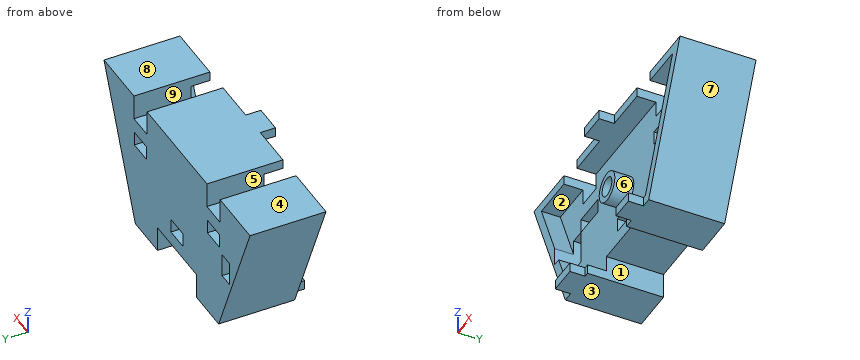
Autodesk Inventor part; units mm, degrees
ref_plane "YZ Plane" through (0, 0, 0) normal (1, 0, 0) x (0, 1, 0)
ref_plane "XZ Plane" through (0, 0, 0) normal (0, 1, 0) x (-1, 0, 0)
ref_plane "XY Plane" through (0, 0, 0) normal (0, 0, 1) x (1, 0, 0)
sketch "Sketch1" plane through (0, 0, 0) normal (0, 1, 0) x (-1, 0, 0)
  line L0 (-15, 7.5) -> (15, 7.5)
  line L1 (15, 7.5) -> (15, -7.5)
  line L2 (15, -7.5) -> (-15, -7.5)
  line L3 (-15, -7.5) -> (-15, 7.5)
  line L4 (-15, 7.5) -> (15, -7.5) construction
  line L5 (15, 7.5) -> (-15, -7.5) construction
  point P0 (0, 0)
  dimension "d0" = 30
  dimension "d1" = 15
extrude "Extrusion1" add sketch "Sketch1" along normal blind 8
sketch "Sketch3" plane through (0, 8, 0) normal (0, 1, 0) x (1, 0, 0)
  line L0 (-15, 7.5) -> (-15, -7.5)
  line L1 (-15, -7.5) -> (15, -7.5)
  line L2 (-15, -7.5) -> (15, -7.5)
  line L3 (15, -7.5) -> (8.5, 7.6369)
  line L4 (-15, -7.5) -> (-8.5, 7.6369)
  line L5 (-8.5, 7.6369) -> (8.5, 7.6369)
  line L6 (-10.75, -1.2417) -> (-9.25, -1.2417)
  line L7 (-9.25, -1.2417) -> (-9.25, 1.2583)
  line L8 (-9.25, 1.2583) -> (-10.75, 1.2583)
  line L9 (-10.75, 1.2583) -> (-10.75, -1.2417)
  line L10 (-10.75, -1.2417) -> (-9.25, 1.2583) construction
  line L11 (-9.25, -1.2417) -> (-10.75, 1.2583) construction
  line L12 (-6.25, -3.25) -> (-8.75, -3.25)
  line L13 (-8.75, -3.25) -> (-8.75, -1.75)
  line L14 (-8.75, -1.75) -> (-6.25, -1.75)
  line L15 (-6.25, -1.75) -> (-6.25, -3.25)
  line L16 (-6.25, -3.25) -> (-8.75, -1.75) construction
  line L17 (-8.75, -3.25) -> (-6.25, -1.75) construction
  line L18 (8.75, -1.75) -> (6.25, -1.75)
  line L19 (6.25, -1.75) -> (6.25, -3.25)
  line L20 (6.25, -3.25) -> (8.75, -3.25)
  line L21 (8.75, -3.25) -> (8.75, -1.75)
  line L22 (8.75, -1.75) -> (6.25, -3.25) construction
  line L23 (6.25, -1.75) -> (8.75, -3.25) construction
  line L24 (15, 7.5) -> (-15, 7.5)
  line L25 (-15, -7.5) -> (-15, 7.5)
  line L26 (-15, 7.5) -> (15, 7.5)
  line L27 (15, 7.5) -> (15, -7.5)
  line L28 (1.25, 1.8869) -> (-1.25, 1.8869)
  line L29 (-1.25, 1.8869) -> (-1.25, 3.3869)
  line L30 (-1.25, 3.3869) -> (1.25, 3.3869)
  line L31 (1.25, 3.3869) -> (1.25, 1.8869)
  line L32 (1.25, 1.8869) -> (-1.25, 3.3869) construction
  line L33 (-1.25, 1.8869) -> (1.25, 3.3869) construction
  point P0 (0, 0)
  point P1 (-10, 0.0083)
  point P2 (-7.5, -2.5)
  point P3 (7.5, -2.5)
  point P4 (0, -7.5)
  point P5 (0, -7.5)
  point P6 (0, 2.6369)
  point P7 (8.5588, 7.5)
  point P8 (-8.5588, 7.5)
  dimension "d19" = 17
  dimension "d20" = 1.5
  dimension "d21" = 2.5
  dimension "d22" = 5
  dimension "d24" = 7.5
  dimension "d25" = 7.5
  dimension "d26" = 5
  dimension "d27" = 5
  dimension "d28" = 5
  dimension "d29" = 0
extrude "Extrusion3" cut sketch "Sketch3" against normal blind 8 contours L24 L4 L0 | L3 L24 L27 | L9 L8 L7 L6 | L12 L13 L14 L15 | L21 L20 L19 L18 | L28 L29 L30 L31
sketch "Sketch4" plane through (0, 0, 0) normal (0, -1, 0) x (1, 0, 0)
  line L0 (-9.25, 1.7417) -> (-10.75, 1.7417)
  line L1 (-10.75, 1.7417) -> (-10.75, -1.7583)
  line L2 (-10.75, -1.7583) -> (-9.25, -1.7583)
  line L3 (-9.25, -1.7583) -> (-9.25, 1.7417)
  line L4 (-9.25, 1.7417) -> (-10.75, -1.7583) construction
  line L5 (-10.75, 1.7417) -> (-9.25, -1.7583) construction
  line L6 (-10.75, -1.2583) -> (-10.75, 1.2417)
  line L7 (-9.25, 1.2417) -> (-9.25, -1.2583)
  line L8 (-9.25, -1.2583) -> (-10.75, -1.2583)
  line L9 (-10.75, 1.2417) -> (-9.25, 1.2417)
  line L10 (-8.75, 3.25) -> (-6.25, 3.25) construction
  line L11 (-7.5, 3.25) -> (-7.5, 1.75) construction
  line L12 (-8.75, 1.75) -> (-6.25, 1.75) construction
  line L13 (-1.25, -1.8869) -> (1.25, -1.8869) construction
  line L14 (0, -1.8869) -> (0, -3.3869) construction
  line L15 (1.25, -3.3869) -> (-1.25, -3.3869) construction
  line L16 (6.25, 3.25) -> (8.75, 3.25) construction
  line L17 (7.5, 3.25) -> (7.5, 1.75) construction
  line L18 (8.75, 1.75) -> (6.25, 1.75) construction
  line L19 (9.25, 3.25) -> (5.75, 3.25)
  line L20 (5.75, 3.25) -> (5.75, 1.75)
  line L21 (5.75, 1.75) -> (9.25, 1.75)
  line L22 (9.25, 1.75) -> (9.25, 3.25)
  line L23 (9.25, 3.25) -> (5.75, 1.75) construction
  line L24 (5.75, 3.25) -> (9.25, 1.75) construction
  line L25 (1.75, -1.8869) -> (-1.75, -1.8869)
  line L26 (-1.75, -1.8869) -> (-1.75, -3.3869)
  line L27 (-1.75, -3.3869) -> (1.75, -3.3869)
  line L28 (1.75, -3.3869) -> (1.75, -1.8869)
  line L29 (1.75, -1.8869) -> (-1.75, -3.3869) construction
  line L30 (-1.75, -1.8869) -> (1.75, -3.3869) construction
  line L31 (-5.75, 3.25) -> (-9.25, 3.25)
  line L32 (-9.25, 3.25) -> (-9.25, 1.75)
  line L33 (-9.25, 1.75) -> (-5.75, 1.75)
  line L34 (-5.75, 1.75) -> (-5.75, 3.25)
  line L35 (-5.75, 3.25) -> (-9.25, 1.75) construction
  line L36 (-9.25, 3.25) -> (-5.75, 1.75) construction
  point P0 (0, 0)
  point P1 (-10, -0.0083)
  point P2 (7.5, 2.5)
  point P3 (0, -2.6369)
  point P4 (-7.5, 2.5)
  point P5 (-10.75, 1.2417)
  dimension "d32" = 0
  dimension "d33" = 0
  dimension "d34" = 0.5
  dimension "d35" = 0.5
  dimension "d36" = 3.5
  dimension "d37" = 3.5
  dimension "d38" = 3.5
extrude "Extrusion4" cut sketch "Sketch4" against normal blind 3.5
sketch "Sketch5" plane through (0, 0, 0) normal (0, -1, 0) x (1, 0, 0)
  line L0 (-9.25, -1.7583) -> (-10.75, -1.7583)
  line L1 (-15, 7.5) -> (-8.5588, -7.5)
  line L2 (8.5588, -7.5) -> (-8.5588, -7.5)
  line L3 (-7.8999, -6.5) -> (7.8999, -6.5)
  line L4 (7.8999, -6.5) -> (13.4823, 6.5)
  line L5 (8.5588, -7.5) -> (15, 7.5)
  line L6 (-15, 7.5) -> (15, 7.5)
  line L7 (13.4823, 6.5) -> (-14, 6.5)
  line L8 (-7.8999, -6.5) -> (-13.4823, 6.5)
  point P0 (0, 0)
  point P1 (-13.4823, 6.5)
  dimension "d41" = 1
  dimension "d42" = 1
  dimension "d43" = 1
  dimension "d44" = 1
  dimension "d45" = 1
  dimension "d46" = 1
sketch "Sketch2" plane through (0, 8, 0) normal (0, 1, 0) x (1, 0, 0)
  line L0 (4, 7.5) -> (-4, 7.5)
  line L1 (-4, 7.5) -> (-4, 4.8)
  line L2 (-4, 4.8) -> (4, 4.8)
  line L3 (4, 4.8) -> (4, 7.5)
  line L4 (4, 7.5) -> (-4, 4.8) construction
  line L5 (-4, 7.5) -> (4, 4.8) construction
  line L6 (-6.15, -4.8) -> (-8.85, -4.8)
  line L7 (-8.85, -4.8) -> (-8.85, -7.5)
  line L8 (-8.85, -7.5) -> (-6.15, -7.5)
  line L9 (-6.15, -7.5) -> (-6.15, -4.8)
  line L10 (-6.15, -4.8) -> (-8.85, -7.5) construction
  line L11 (-8.85, -4.8) -> (-6.15, -7.5) construction
  line L12 (8.85, -4.8) -> (6.15, -4.8)
  line L13 (6.15, -4.8) -> (6.15, -7.5)
  line L14 (6.15, -7.5) -> (8.85, -7.5)
  line L15 (8.85, -7.5) -> (8.85, -4.8)
  line L16 (8.85, -4.8) -> (6.15, -7.5) construction
  line L17 (6.15, -4.8) -> (8.85, -7.5) construction
  point P0 (0, 0)
  point P1 (0, 6.15)
  point P2 (-7.5, -6.15)
  point P3 (7.5, -6.15)
  dimension "d8" = 8
  dimension "d9" = 2.7
  dimension "d10" = 7.5
  dimension "d11" = 2.7
  dimension "d12" = 7.5
  dimension "d13" = 7.5
  dimension "d15" = 7.5
  dimension "d16" = 7.5
extrude "Extrusion2" cut sketch "Sketch2" against normal blind 8
extrude "Extrusion5" cut sketch "Sketch5" against normal blind 2 contours L8 L7 L4 L3
sketch "Sketch6" plane through (0, 2, 0) normal (0, -1, 0) x (1, 0, 0)
  circle A0 centre (0, 0) radius 1
  circle A1 centre (0, 0) radius 1.6
  dimension "d49" = 2
  dimension "d50" = 0.6
extrude "Extrusion6" add sketch "Sketch6" along normal blind 2
sketch "Sketch7" plane through (0, 0, 0) normal (0, -1, 0) x (1, 0, 0)
  circle A0 centre (0, 0) radius 1
  dimension "d74" = 2
extrude "Extrusion7" cut sketch "Sketch7" against normal blind 5
sketch "Sketch8" plane through (0, 0, 0) normal (0, -1, 0) x (1, 0, 0)
  line L0 (-7.5, -7.5) -> (-4.5, -7.5)
  line L1 (-4.5, -7.5) -> (-4.5, -6.5)
  line L2 (-4.5, -6.5) -> (-7.5, -6.5)
  line L3 (-7.5, -6.5) -> (-7.5, -7.5)
  line L4 (7.5, -6.5) -> (5, -6.5)
  line L5 (5, -6.5) -> (5, -7.5)
  line L6 (5, -7.5) -> (7.5, -7.5)
  line L7 (7.5, -7.5) -> (7.5, -6.5)
  line L8 (1.5, 7.5) -> (-1.5, 7.5)
  line L9 (-1.5, 7.5) -> (-1.5, 6.5)
  line L10 (-1.5, 6.5) -> (1.5, 6.5)
  line L11 (1.5, 6.5) -> (1.5, 7.5)
  line L12 (1.5, 7.5) -> (-1.5, 6.5) construction
  line L13 (-1.5, 7.5) -> (1.5, 6.5) construction
  point P0 (0, 0)
  point P1 (0, 7)
  point P2 (-6, -6.5)
  point P3 (6.25, -7.5)
  point P4 (-6, -7.5)
  dimension "d55" = 3
  dimension "d56" = 1
  dimension "d57" = 2.5
  dimension "d58" = 1
  dimension "d59" = 3
  dimension "d60" = 1
  dimension "d62" = 7.5
  dimension "d63" = 7.5
  dimension "d64" = 7.5
  dimension "d72" = 9.5
  dimension "d73" = 6
extrude "Extrusion8" add sketch "Sketch8" along normal blind 1.6
properties part number "MUX"
For this review, take the finished solid that the model builds, in its own axes (mm). Face numbers are marked on the shaded views. A direction names the side the tool comes from. Round coordinates to 2 decimals unless told otherwise and drop trailing zeros. Loops run counter-clockwise (first coordinate to the right, second up) from the corner with the lowest first, then second, coordinate; pieces in that order, holes last.
Q1. Machinability: for the marked faces 1, 2, 3, 4 and 5, which of the approach directions +Z, -Z, +X, -X, +Y, -Y give a long, thin tool a straight path to every point of the face, cutting with its end or side? Answer none if there is none.
Result sheet:
face 1: -Z, +Y, -Y
face 2: -Y
face 3: -Z, +X, -X, +Y, -Y
face 4: +Z, +X, -X, +Y, -Y
face 5: +Z, +Y, -Y
Q2. Insertion check: pin 1 Ø1.1 at (y, z) = (-1, 7) entering from +X; pin 2 Ø2 at (x, y) = (-8.5, 0.5) entering from +Z; pin 3 Ø1.6 at (y, z) = (5.5, -2.5) entering from -X; pin 4 Ø3 at (y, z) = (3.5, 6.5) entering from +X. Each pin has a flat end and moves straight along its axis. Give the tip position at first contact, or say it passes through.
Result sheet:
pin 1: stops at x = 1.5
pin 2: stops at z = 7.5
pin 3: stops at x = -11.05
pin 4: stops at x = 15
Q3. Add section B-B on x = 0. Write out the cut boundary in (y, z), plus the area to 3 significant figures.
Result sheet:
outline: (-1.6, 6.5) - (2, 6.5) - (2, 1.6) - (0, 1.6) - (0, 1) - (5, 1) - (5, -1) - (0, -1) - (0, -1.6) - (2, -1.6) - (2, -1.89) - (8, -1.89) - (8, 7.5) - (-1.6, 7.5) - close; (2, -4.8) - (8, -4.8) - (8, -3.39) - (2, -3.39) - close
area: 64.8 mm2
Q4. Mouldability with a two-part tool opening along Z and no side actions: class the marked faces 6, 7, 8 and 9 as +Z half, -Z half, draft (parallel to the pull), parting line (faces both ways), or undercut.
Result sheet:
face 6: undercut
face 7: -Z half
face 8: +Z half
face 9: draft
Q5. Add section C-C on y = 6.5. Give the number of separate pieces and of enclosed holes in the cut face, plus the area to 3 significant figures.
Result sheet:
separate pieces: 1
enclosed holes: 4
area: 302 mm2
Q6. Add section A-A on y = 1.25. Write out the cut boundary in (x, z).
Result sheet:
outline: (-15, 7.5) - (-8.56, -7.5) - (-4, -7.5) - (-4, -6.5) - (-7.9, -6.5) - (-9.94, -1.76) - (-10.75, -1.76) - (-10.75, 0.14) - (-13.48, 6.5) - (-8.85, 6.5) - (-8.85, 7.5) - close; (-6.15, 6.5) - (6.15, 6.5) - (6.15, 7.5) - (-6.15, 7.5) - close; circle Ø3.2 at (0, 0); (4, -7.5) - (8.56, -7.5) - (15, 7.5) - (8.85, 7.5) - (8.85, 6.5) - (13.48, 6.5) - (7.9, -6.5) - (4, -6.5) - close; hole circle Ø2 at (0, 0)
Q7. To check wall thickness, follow line 1 along Z through (x, y) = (0, 3.8); line 2 along Z through (x, y) = (0, 1.05); line 3 along X through (y, z) = (6.25, 2.75). State the ranges of each line that lie inside material, in increasing order.
Result sheet:
line 1: z = -4.8 to -3.39, -1.89 to -1, 1 to 7.5
line 2: z = -1.6 to -1, 1 to 1.6, 6.5 to 7.5
line 3: x = -12.96 to -8.75, -6.25 to 6.25, 8.75 to 12.96
